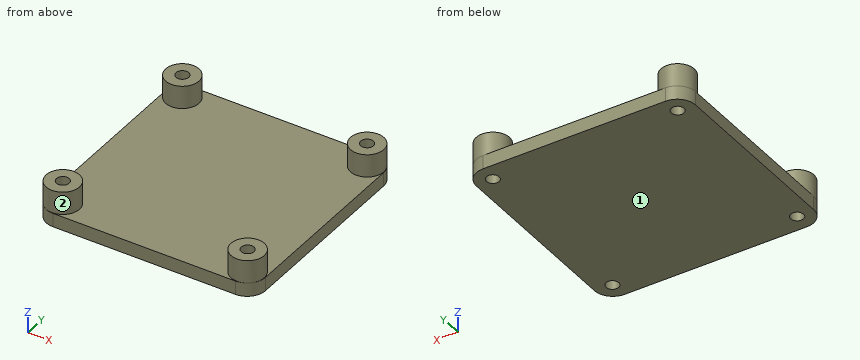
```python
from build123d import *

# Parameters (mm, degrees)
SKETCH_1_W          = 48
SKETCH_1_H          = 48
SKETCH_1_R          = 1.4
EXTRUDE_1_DEPTH     = 3
FILLET_1_R          = 4
SKETCH_2_R          = 3.646446609
EXTRUDE_2_DEPTH     = 5
SKETCH_3_R          = 1.4
CUT_EXTRUDE_1_DEPTH = 99


with BuildPart() as part:
    # 草图1 → 凸台-拉伸1 (new body)
    with BuildSketch(Plane.XY):
        Rectangle(SKETCH_1_W, SKETCH_1_H)
        with Locations((-20.25, 20.25)):
            Circle(SKETCH_1_R, mode=Mode.SUBTRACT)
        with Locations((20.25, 20.25)):
            Circle(SKETCH_1_R, mode=Mode.SUBTRACT)
        with Locations((20.25, -20.25)):
            Circle(SKETCH_1_R, mode=Mode.SUBTRACT)
        with Locations((-20.25, -20.25)):
            Circle(SKETCH_1_R, mode=Mode.SUBTRACT)
    extrude(amount=EXTRUDE_1_DEPTH)

    # 圆角1
    fillet_1_edges = [part.edges().sort_by_distance(p)[0] for p in [
        (24, -24, 1.5),
        (-24, -24, 1.5),
        (-24, 24, 1.5),
        (24, 24, 1.5),
    ]]
    fillet(fillet_1_edges, radius=FILLET_1_R)

    # 草图2 → 凸台-拉伸2 (add)
    with BuildSketch(Plane.XY.offset(3)):
        with Locations(Location((-20.25, 20.25, 0), (0, 0, 134.998572702))):
            Circle(SKETCH_2_R)
        with Locations(Location((20.25, 20.25, 0), (0, 0, 44.998572702))):
            Circle(SKETCH_2_R)
        with Locations(Location((20.25, -20.25, 0), (0, 0, 314.998572702))):
            Circle(SKETCH_2_R)
        with Locations(Location((-20.25, -20.25, 0), (0, 0, 224.998572702))):
            Circle(SKETCH_2_R)
    extrude(amount=EXTRUDE_2_DEPTH)

    # 草图3 → 切除-拉伸1 (cut)
    with BuildSketch(Plane(origin=(0, 0, 0), x_dir=(-1, 0, 0), z_dir=(0, 0, -1))):
        with Locations(Location((-20.25, 20.25, 0), (0, 0, 180))):
            Circle(SKETCH_3_R)
        with Locations(Location((20.25, 20.25, 0), (0, 0, 180))):
            Circle(SKETCH_3_R)
        with Locations(Location((20.25, -20.25, 0), (0, 0, 180))):
            Circle(SKETCH_3_R)
        with Locations(Location((-20.25, -20.25, 0), (0, 0, 180))):
            Circle(SKETCH_3_R)
    extrude(amount=-CUT_EXTRUDE_1_DEPTH, mode=Mode.SUBTRACT)


solid = part.part
```
Here's how the part is built. I have some questions about the finished solid (model axes, mm). Face numbers are marked on the shaded views. Coordinates: 2 decimals unless noted, no trailing zeros. Loops run counter-clockwise (first coordinate to the right, second up) from the corner with the lowest first, then second, coordinate; pieces in that order, holes last. Notation, with made-up numbers: M -2,-22.75 L 34,-22.75 A15 cw 34,-14.75 Z; hole C -40,68.5 d7. An arc over 180 degrees is marked long. One line per item, written item: value.
1. Thinking about a two-plate mould opening in X: for the marked faces 1 and 2, which applies, +X half, -X half, draft (parallel to the pull), parting line (faces both ways), or undercut?
Geometry says:
face 1: draft
face 2: undercut
2. Will these pins go through, and if not, where does the flat tip stop? pin 1 Ø12 at (x, y) = (10.5, -4.5) entering from -Z; pin 2 Ø12 at (x, y) = (3.5, 6.5) entering from +Z; pin 3 Ø1.5 at (x, z) = (18, 6) entering from +Y.
Geometry says:
pin 1: stops at z = 0
pin 2: stops at z = 3
pin 3: stops at y = 23.57
3. Imagine slicing it at D-D (x = -18). List the corners of the cut face in (y, z) for me.
Geometry says:
outline: M -24,0 L 24,0 L 24,3 L 23.12,3 L 23.12,8 L 17.38,8 L 17.38,3 L -17.38,3 L -17.38,8 L -23.12,8 L -23.12,3 L -24,3 Z
4. Imagine slicing it at A-A (z = 4). List the corners of the cut face in (x, y) for me.
Geometry says:
outline: C -20.25,-20.25 d7.29; C -20.25,20.25 d7.29; C 20.25,-20.25 d7.29; C 20.25,20.25 d7.29; hole C -20.25,-20.25 d2.8; hole C -20.25,20.25 d2.8; hole C 20.25,-20.25 d2.8; hole C 20.25,20.25 d2.8
5. Imagine slicing it at B-B (x = -8). List the corners of the cut face in (y, z) for me, and give its area (3 significant figures).
Geometry says:
outline: M -24,0 L 24,0 L 24,3 L -24,3 Z
area: 144 mm2
6. Please list where these lines run through material, in increasing order: probe 1 along Y at (x, z) = (20.25, 1.2); probe 2 along Y at (x, z) = (20.25, 6.35).
Geometry says:
probe 1: y = -23.99 to -21.65, -18.85 to 18.85, 21.65 to 23.99
probe 2: y = -23.9 to -21.65, -18.85 to -16.6, 16.6 to 18.85, 21.65 to 23.9
